CAD build for the part. Positions are in the model's coordinates, mm. Face numbers are marked on the shaded views. Give positions to 0.01 mm unless a question says otherwise; leave off trailing zeros. Loops run counter-clockwise (first coordinate to the right, second up) from the corner with the lowest first, then second, coordinate; pieces in that order, holes last. Notation, with made-up numbers: M -13.5,-30.75 L 9.5,-30.75 A9 cw 9.5,-21.75 Z; hole C 36,23 d7. An arc over 180 degrees is marked long. Answer as CSV lines item,"result".
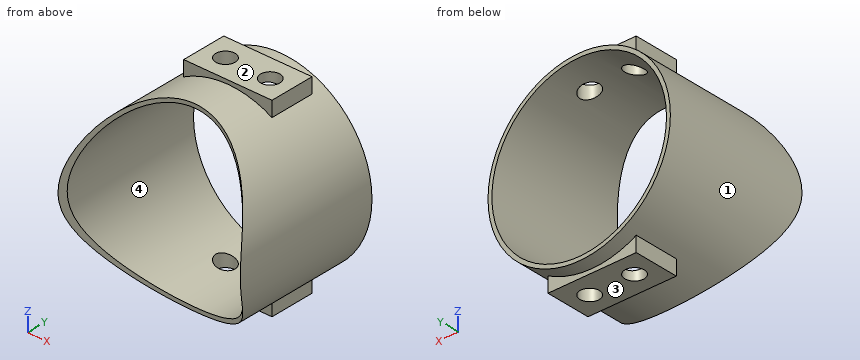
Autodesk Inventor part; units mm, degrees
ref_plane "YZ Plane" through (0, 0, 0) normal (1, 0, 0) x (0, 1, 0)
ref_plane "XZ Plane" through (0, 0, 0) normal (0, 1, 0) x (-1, 0, 0)
sketch "Sketch1" plane through (0, 0, 0) normal (0, 1, 0) x (-1, 0, 0)
  circle A0 centre (20.8145, -14.703) radius 14.1152
  circle A1 centre (20.8145, -14.703) radius 13.5152
  point P0 (0, 0)
  dimension "d0" = 0.6
extrude "Extrusion1" add sketch "Sketch1" along normal blind 24
ref_plane "Work Plane1" through (0, 0, -29) normal (0, 0, 1) x (1, 0, 0)
sketch "Sketch3" plane through (0, 0, 0) normal (1, 0, 0) x (0, 1, 0)
  point P0 (0, 0)
sketch "Sketch4" plane through (0, 0, 0) normal (0, 0, 1) x (1, 0, 0)
  line L0 (-34.9297, 0) -> (-34.9297, 24)
  line L1 (-6.6992, 0) -> (-6.6992, 24)
  line L2 (-34.9297, 18.2399) -> (-20.8145, 18.2399) construction
  line L3 (-20.8145, 18.2399) -> (-6.6992, 18.2399) construction
  line L4 (-13.9813, 14.7399) -> (-27.6476, 14.7399)
  line L5 (-27.6476, 14.7399) -> (-27.6476, 21.7399)
  line L6 (-27.6476, 21.7399) -> (-13.9813, 21.7399)
  line L7 (-13.9813, 21.7399) -> (-13.9813, 14.7399)
  line L8 (-13.9813, 14.7399) -> (-27.6476, 21.7399) construction
  line L9 (-27.6476, 14.7399) -> (-13.9813, 21.7399) construction
  point P0 (0, 0)
  dimension "d14" = 7
extrude "Extrusion3" add sketch "Sketch4" against normal up to surface
sketch "Sketch5" plane through (-20.8145, 24, -14.703) normal (0, 1, 0) x (1, 0, 0)
  point P0 (20.8145, -14.703)
  point P1 (0, 0)
ref_plane "Work Plane2" through (-20.8145, 24, -14.703) normal (0, 0, 1) x (1, 0, 0)
mirror "Mirror1" about plane through (-20.8145, 24, -14.703) normal (0, 0, 1) of "Extrusion3"
sketch "Sketch6" plane through (0, 0, 0) normal (0, 0, 1) x (1, 0, 0)
  line L0 (-13.9813, 14.7399) -> (-13.9813, 21.7399)
  line L1 (-13.9813, 21.7399) -> (-27.6476, 21.7399)
  line L2 (-27.6476, 21.7399) -> (-27.6476, 14.7399)
  line L3 (-27.6476, 14.7399) -> (-13.9813, 14.7399)
  line L4 (-17.3456, 21.7399) -> (-17.3456, 18.2399) construction
  line L5 (-17.3456, 18.2399) -> (-17.3456, 14.7399) construction
  line L6 (-24.2833, 21.7399) -> (-24.2833, 18.2399) construction
  line L7 (-24.2833, 18.2399) -> (-24.2833, 14.7399) construction
  line L8 (-17.3456, 18.2399) -> (-13.9813, 18.2399) construction
  line L9 (-13.9813, 21.7399) -> (-13.9813, 14.7399) construction
  line L10 (-24.2833, 18.2399) -> (-27.6476, 18.2399) construction
  circle A0 centre (-17.3456, 18.2399) radius 1.5
  circle A1 centre (-24.2833, 18.2399) radius 1.5
  point P0 (0, 0)
  dimension "d10" = 3
  dimension "d11" = 3
extrude "Extrusion4" cut sketch "Sketch6" against normal blind 72.25 contours A0 | A1
sketch "Sketch7" plane through (0, 0, 0) normal (0, 0, 1) x (1, 0, 0)
  circle A0 centre (-20.8145, -7.4962) radius 16.4655
  line L0 (-34.9297, 0) -> (-34.9297, 24)
  line L1 (-6.6992, 0) -> (-6.6992, 24)
  line L2 (-34.9297, 12) -> (-20.8145, 12)
  line L3 (-20.8145, 12) -> (-6.6992, 12)
  line L4 (-20.8145, 12) -> (-20.8145, -15.8986) construction
  point P0 (0, 0)
  dimension "d15" = 32.931
extrude "Extrusion5" cut sketch "Sketch7" against normal blind 60.25 contours A0
Q1. Cut at C-C (y = 19). Write the cut outline in (x, z).
Solution:
outline,"M -27.65,-29.41 L -25.58,-29.41 L -25.58,-27.35 A13.52 cw -25.58,-2.05 L -25.58,0 L -27.65,0 L -27.65,-2.35 A14.12 ccw -27.65,-27.05 Z; M -22.99,-29.41 L -18.64,-29.41 L -18.64,-28.04 A13.52 cw -22.99,-28.04 Z; M -22.99,-1.36 A13.52 cw -18.64,-1.36 L -18.64,0 L -22.99,0 Z; M -16.05,-29.41 L -13.98,-29.41 L -13.98,-27.05 A14.12 ccw -13.98,-2.35 L -13.98,0 L -16.05,0 L -16.05,-2.05 A13.52 cw -16.05,-27.35 Z"
Q2. Wall check: line 1 (X direction, y = 8.5, z = -14.5); line 2 (X direction, y = 11.25, z = -23.25); line 3 (Z direction, x = -11.5, y = 21.5). Give the ranges that are in metal, low to high. Write a range as [from, to].
Solution:
line 1,"x = [-34.93, -34.33], [-7.3, -6.7]"
line 2,"x = [-32.05, -31.28], [-10.35, -9.58]"
line 3,"z = [-25.31, -24.5], [-4.91, -4.1]"
Q3. Cut at B-B (z = -8.5). Write the cut outline in (x, y).
Solution:
outline,"M -33.49,3.01 A16.47 cw -32.82,3.77 L -32.82,24 L -33.49,24 Z; M -8.81,3.77 A16.47 cw -8.14,3.01 L -8.14,24 L -8.81,24 Z"
Q4. Cut at A-A (y = 6). Write the cut outline in (x, z), and give its area (3 significant figures).
Solution:
outline,"M -30.25,-25.2 L -30.25,-24.38 A13.52 cw -30.25,-5.02 L -30.25,-4.2 A14.12 ccw Z; M -11.38,-25.2 A14.12 ccw -11.38,-4.2 L -11.38,-5.02 A13.52 cw -11.38,-24.38 Z"
area,"27.2 mm²"
Q5. Mould opens along Z. For the marked faces 1, 2, 3 and 4 say: released by +Z, released by -Z, zero draft, split by the parting line, or undercut.
Solution:
face 1,"split by the parting line"
face 2,"released by +Z"
face 3,"released by -Z"
face 4,"undercut"
Q6. Pin check, flat tips, straight feed: P1, Ø2, axis at y = 14, z = -13, coming from the +X side; P2, Ø3, axis at y = 15, z = -22.5, coming from the +X side; P3, Ø5, axis at x = -31, y = 6.5, coming from the +Z side; P4, Ø1.8, axis at x = -24.28, y = 18.24, coming from the -Z side. Stop position of each tip, or through.
Solution:
P1,"stops at x = -6.72"
P2,"stops at x = -8.18"
P3,"stops at z = -2.9"
P4,"passes through"
Q7. Cut at D-D (x = -18.25). Write the cut outline in (y, z).
Solution:
outline,"M 8.77,-28.58 L 14.74,-28.58 L 14.74,-29.41 L 17.04,-29.41 L 17.04,-27.97 L 8.77,-27.97 Z; M 8.77,-1.43 L 17.04,-1.43 L 17.04,0 L 14.74,0 L 14.74,-0.82 L 8.77,-0.82 Z; M 19.44,-29.41 L 21.74,-29.41 L 21.74,-28.58 L 24,-28.58 L 24,-27.97 L 19.44,-27.97 Z; M 19.44,-1.43 L 24,-1.43 L 24,-0.82 L 21.74,-0.82 L 21.74,0 L 19.44,0 Z"
